```python
from build123d import *

# Parameters (mm, degrees)
SKETCH1_W               = 25.6
SKETCH1_H               = 17.7
BOSS_EXTRUDE1_DEPTH     = 4.6
FILLET1_R               = 2.5
SKETCH3_R               = 1.5
CUT_EXTRUDE1_DEPTH      = 32.461246002
MIRROR2_COPY_1_SKETCH_R = 1.5
MIRROR2_COPY_1_DEPTH    = 32.461246002
SKETCH6_W               = 3.5
SKETCH6_H               = 4
BOSS_EXTRUDE2_DEPTH     = 2.5


with BuildPart() as part:
    # Sketch1 → Boss-Extrude1 (new body)
    with BuildSketch(Plane(origin=(0, 0, 0), x_dir=(1, 0, 0), z_dir=(0, 1, 0))):
        with Locations((12.8, 8.85)):
            Rectangle(SKETCH1_W, SKETCH1_H)
    extrude(amount=BOSS_EXTRUDE1_DEPTH)

    # Fillet1
    fillet1_edges = [part.edges().sort_by_distance(p)[0] for p in [
        (0, 2.3, -17.7),
        (0, 2.3, 0),
        (25.6, 2.3, 0),
        (25.6, 2.3, -17.7),
    ]]
    fillet(fillet1_edges, radius=FILLET1_R)

    # Sketch3 → Cut-Extrude1 (cut, through all)
    with BuildSketch(Plane(origin=(0, 4.6, 0), x_dir=(1, 0, 0), z_dir=(0, 1, 0))):
        with Locations(Location((2.603725991, 3.494605911, 0), (0, 0, 270))):
            Circle(SKETCH3_R)
    cut_extrude1 = extrude(amount=-CUT_EXTRUDE1_DEPTH, mode=Mode.SUBTRACT)

    # Mirror1: Cut-Extrude1 across plane
    add(cut_extrude1.mirror(Plane.XY.offset(-8.85)), mode=Mode.SUBTRACT)

    # Mirror2: Cut-Extrude1 across plane
    add(cut_extrude1.mirror(Plane.ZY.offset(-12.8)), mode=Mode.SUBTRACT)

    # Mirror2 copy 1 sketch → Mirror2 copy 1 (cut, through all)
    with BuildSketch(Plane(origin=(25.6, 4.6, -17.7), x_dir=(-1, 0, 0), z_dir=(0, 1, 0))):
        with Locations(Location((2.603725991, 3.494605911, 0), (0, 0, 270))):
            Circle(MIRROR2_COPY_1_SKETCH_R)
    extrude(amount=-MIRROR2_COPY_1_DEPTH, mode=Mode.SUBTRACT)

    # Sketch6 → Boss-Extrude2 (add)
    with BuildSketch(Plane(origin=(0, 4.6, 0), x_dir=(1, 0, 0), z_dir=(0, 1, 0))):
        with Locations((1.75, 8.705394089)):
            Rectangle(SKETCH6_W, SKETCH6_H)
    boss_extrude2 = extrude(amount=BOSS_EXTRUDE2_DEPTH)

    # Mirror3: Boss-Extrude2 across plane
    add(boss_extrude2.mirror(Plane.ZY.offset(-12.8)))


solid = part.part
```
Input: part model. Units: mm. Frame: model coordinates. A direction names the side the tool comes from. Give positions to 0.01 mm unless a question says otherwise; leave off trailing zeros. Order: outer loops, then holes, each group sorted by start corner. A loop starts at its lowest first (then second) coordinate and runs counter-clockwise, first axis right, second up. Notation, with made-up numbers: M 53.5,42 L 105.5,42 A10 cw 105.5,50 Z; hole C 82.5,34 d10. An arc over 180 degrees is marked long. Return JSON: item names as keys, results as strings.
Item 1: Cut plane C-C (x = 24). Return loops of the section in (y, z).
Solutions:
{"outline": "M 0,-17.53 L 4.6,-17.53 L 4.6,-15.32 L 0,-15.32 Z; M 0,-13.09 L 4.6,-13.09 L 4.6,-10.71 L 7.1,-10.71 L 7.1,-6.71 L 4.6,-6.71 L 4.6,-4.61 L 0,-4.61 Z; M 0,-2.38 L 4.6,-2.38 L 4.6,-0.17 L 0,-0.17 Z"}
Item 2: Cut plane A-A (y = 5.75). Return loops of the section in (x, z).
Solutions:
{"outline": "M 0,-10.71 L 3.5,-10.71 L 3.5,-6.71 L 0,-6.71 Z; M 22.1,-10.71 L 25.6,-10.71 L 25.6,-6.71 L 22.1,-6.71 Z"}
Item 3: Access query for faces 1 (the cylindrical face through (23.909, 2.332, -13.015)), 2 (the flat face through (3.5, 6, -9)), 3 (the flat face through (24, 6, -10.705)), 4 (the flat face through (2, 6, -6.705)). Directions: +Z, -Z, +X, -X, +Y, -Y. A direction counts if a zero-diameter tool reaches every point of the face in a straight line with its end or side. Return the directions, or none.
Solutions:
{"face 1": "+Y, -Y", "face 2": "+Z, -Z, +Y", "face 3": "-Z, +X, -X, +Y", "face 4": "+Z, +X, -X, +Y"}
Item 4: First-contact query: P1, Ø0.8, axis at x = 23, y = 6, coming from the +Z side; P2, Ø1.2, axis at x = 24, y = 6.5, coming from the -Z side; P3, Ø5, axis at x = 18.5, z = -15.5, coming from the +Y side; P4, Ø2.5, axis at x = 2.6, z = -3.49, coming from the +Y side. Flat tips, straight axial feed; report the tip coordinate or a pass-through.
Solutions:
{"P1": "z = -6.71", "P2": "z = -10.71", "P3": "y = 4.6", "P4": "through"}
Item 5: Cut plane B-B (z = -4.25). Return loops of the section in (x, y), then the cut area to 3 significant figures.
Solutions:
{"outline": "M 0,0 L 1.31,0 L 1.31,4.6 L 0,4.6 Z; M 3.9,0 L 21.7,0 L 21.7,4.6 L 3.9,4.6 Z; M 24.29,0 L 25.6,0 L 25.6,4.6 L 24.29,4.6 Z", "area": "93.9 mm^2"}
Item 6: Pull-direction query (Z, two-part tool) for faces 5 (the cylindrical face through (24.887, 2.332, -16.948)), 6 (the cylindrical face through (24.848, 2.332, -0.713)), 7 (the cylindrical face through (1.691, 2.332, -13.015)); classes: +Z half, -Z half, draft (parallel to the pull), parting line (faces both ways), or undercut.
Solutions:
{"face 5": "-Z half", "face 6": "+Z half", "face 7": "undercut"}
Item 7: Cut plane D-D (z = -9.5). Return loops of the section in (x, y), then the cut area to 3 significant figures.
Solutions:
{"outline": "M 0,0 L 25.6,0 L 25.6,7.1 L 22.1,7.1 L 22.1,4.6 L 3.5,4.6 L 3.5,7.1 L 0,7.1 Z", "area": "135 mm^2"}
Item 8: Ray query, probe 1 along X at (y, z) = (3.25, -15.25); probe 2 along X at (y, z) = (2.75, -13.75); probe 3 along Z at (x, y) = (3.5, 4). Return the intervals inside material, ascending.
Solutions:
{"probe 1": "0 to 1.53, 3.68 to 21.92, 24.07 to 25.6", "probe 2": "0 to 1.17, 4.03 to 21.57, 24.43 to 25.6", "probe 3": "-17.7 to -15.41, -13 to -4.7, -2.29 to 0"}
